```python
from build123d import *

# Parameters (mm, degrees)
EXTRU_MINCE3_DEPTH       = 85
EXTRU_MINCE4_DEPTH       = 14
ESQUISSE3_W              = 1
ESQUISSE3_H              = 39.023056592
EXTRU_MINCE5_DEPTH       = 14
ESQUISSE4_W              = 1
ESQUISSE4_H              = 39
EXTRU_MINCE6_DEPTH       = 14
ESQUISSE5_W              = 1
ESQUISSE5_H              = 37
EXTRU_MINCE7_DEPTH       = 14
ESQUISSE6_W              = 1
ESQUISSE6_H              = 37
EXTRU_MINCE8_DEPTH       = 14
ESQUISSE9_W              = 26
ESQUISSE9_H              = 39.023056592
ESQUISSE9_H_2            = 39
ESQUISSE9_W_2            = 27
BOSS_EXTRU_2_DEPTH       = 1
CONG_1_R                 = 10
CONG_2_R                 = 10
CONG_3_R                 = 10
CONG_4_R                 = 10
ESQUISSE10_W             = 23
ESQUISSE10_H             = 14
BOSS_EXTRU_3_DEPTH       = 3
ESQUISSE11_W             = 23
ESQUISSE11_H             = 14
BOSS_EXTRU_4_DEPTH       = 3
ESQUISSE14_R             = 1
ENL_V_MAT_EXTRU_2_DEPTH  = 15
ENL_V_START              = -15
ESQUISSE15_R             = 1
ENL_V_MAT_EXTRU_4_DEPTH  = 15
CHANFREIN2_SIZE2         = 1.154700538
CHANFREIN2_SIZE          = 2
CHANFREIN4_SIZE          = 2
CHANFREIN4_SIZE_2        = 2.22122503
BOSS_EXTRU_8_DEPTH       = 2
BOSS_EXTRU_9_DEPTH       = 2
ESQUISSE23_W             = 20
ESQUISSE23_H             = 10
ENL_V_MAT_EXTRU_7_DEPTH  = 2
ESQUISSE24_W             = 20
ESQUISSE24_H             = 10
ENL_V_MAT_EXTRU_9_DEPTH  = 2
ESQUISSE25_W             = 20
ESQUISSE25_H             = 10
ENL_V_MAT_EXTRU_11_DEPTH = 2
ESQUISSE26_W             = 20
ESQUISSE26_H             = 10
ENL_V_MAT_EXTRU_13_DEPTH = 2
ESQUISSE28_W             = 18
ESQUISSE28_H             = 4
R_VOL_MINCE9_ANGLE       = 50
ESQUISSE29_W             = 18
ESQUISSE29_H             = 4
R_VOL_MINCE10_ANGLE      = 50
ESQUISSE31_W             = 18
ESQUISSE31_H             = 4
R_VOL_MINCE11_ANGLE      = 50
ESQUISSE32_W             = 18
ESQUISSE32_H             = 4
R_VOL_MINCE12_ANGLE      = 50


# Some blends are built 0.0001 mm under size
with BuildPart() as part:
    # Esquisse1 → Extru.-Mince3 (new body)
    with BuildSketch(Plane.XY):
        Polygon((37.759483403, 45), (0, 0), (-200, 0), (-237.759483403, 45), (-236.227394517, 46.285575219), (-199.067384684, 2), (-0.932615316, 2), (36.227394517, 46.285575219), align=None)
    extrude(amount=EXTRU_MINCE3_DEPTH)

    # Esquisse2 → Extru.-Mince4 (add)
    with BuildSketch(Plane(origin=(0, 0, 0), x_dir=(-1, 0, 0), z_dir=(0, -1, 0))):
        Polygon((199.067384684, -46), (174, -46), (174, -85), (176, -85), (176, -48), (199.067384684, -48), align=None)
        Polygon((0, -48), (24, -48), (24, -85), (26, -85), (26, -46), (0, -46), align=None)
        Polygon((88.5, -85), (88.5, -48), (111.5, -48), (111.5, -85), (113.5, -85), (113.5, -46), (86.5, -46), (86.5, -85), align=None)
        Polygon((199.067384684, -37), (176, -37), (176, 0), (174, 0), (174, -39), (199.067384684, -39), align=None)
        Polygon((111.5, 0), (111.5, -37), (88.5, -37), (88.5, 0), (86.5, 0), (86.5, -39), (113.5, -39), (113.5, 0), align=None)
        Polygon((0, -39), (26, -39), (26, 0), (24, 0), (24, -37), (0, -37), align=None)
    extrude(amount=EXTRU_MINCE4_DEPTH)

    # Esquisse3 → Extru.-Mince5 (add)
    with BuildSketch(Plane(origin=(0, 0, 0), x_dir=(-1, 0, 0), z_dir=(0, -1, 0))):
        with Locations((199.5, -19.511528296)):
            Rectangle(ESQUISSE3_W, ESQUISSE3_H)
    extrude(amount=EXTRU_MINCE5_DEPTH)

    # Esquisse4 → Extru.-Mince6 (add)
    with BuildSketch(Plane.XZ):
        with Locations((-199.5, 65.5)):
            Rectangle(ESQUISSE4_W, ESQUISSE4_H)
    extrude(amount=EXTRU_MINCE6_DEPTH)

    # Esquisse5 → Extru.-Mince7 (add)
    with BuildSketch(Plane(origin=(0, 0, 0), x_dir=(-1, 0, 0), z_dir=(0, -1, 0))):
        with Locations((0.5, -18.5)):
            Rectangle(ESQUISSE5_W, ESQUISSE5_H)
    extrude(amount=EXTRU_MINCE7_DEPTH)

    # Esquisse6 → Extru.-Mince8 (add)
    with BuildSketch(Plane(origin=(0, 0, 0), x_dir=(-1, 0, 0), z_dir=(0, -1, 0))):
        with Locations((0.5, -66.5)):
            Rectangle(ESQUISSE6_W, ESQUISSE6_H)
    extrude(amount=EXTRU_MINCE8_DEPTH)

    # Esquisse9 → Boss.-Extru.2 (add)
    with BuildSketch(Plane(origin=(0, -14, 0), x_dir=(-1, 0, 0), z_dir=(0, -1, 0))):
        with Locations((187, -19.511528296)):
            Rectangle(ESQUISSE9_W, ESQUISSE9_H)
        with Locations((187, -65.5)):
            Rectangle(ESQUISSE9_W, ESQUISSE9_H_2)
        with Locations((100, -65.5)):
            Rectangle(ESQUISSE9_W_2, ESQUISSE9_H_2)
        with Locations((100, -19.5)):
            Rectangle(ESQUISSE9_W_2, ESQUISSE9_H_2)
        with Locations((13, -65.5)):
            Rectangle(ESQUISSE9_W, ESQUISSE9_H_2)
        with Locations((13, -19.5)):
            Rectangle(ESQUISSE9_W, ESQUISSE9_H_2)
    extrude(amount=BOSS_EXTRU_2_DEPTH)

    # Congé1
    cong_1_edges = [part.edges().sort_by_distance(p)[0] for p in [
        (-100, -15, 39),
    ]]
    fillet(cong_1_edges, radius=CONG_1_R)

    # Congé2
    cong_2_edges = [part.edges().sort_by_distance(p)[0] for p in [
        (-100, -14, 37),
    ]]
    fillet(cong_2_edges, radius=CONG_2_R)

    # Congé3
    cong_3_edges = [part.edges().sort_by_distance(p)[0] for p in [
        (-100, -15, 46),
    ]]
    fillet(cong_3_edges, radius=CONG_3_R)

    # Congé4
    cong_4_edges = [part.edges().sort_by_distance(p)[0] for p in [
        (-100, -14, 48),
    ]]
    fillet(cong_4_edges, radius=CONG_4_R)

    # Esquisse10 → Boss.-Extru.3 (add)
    with BuildSketch(Plane.XY.offset(85)):
        with Locations((-100, -7)):
            Rectangle(ESQUISSE10_W, ESQUISSE10_H)
    extrude(amount=-BOSS_EXTRU_3_DEPTH)

    # Esquisse11 → Boss.-Extru.4 (add)
    with BuildSketch(Plane(origin=(0, 0, 0), x_dir=(-1, 0, 0), z_dir=(0, 0, -1))):
        with Locations((100, -7)):
            Rectangle(ESQUISSE11_W, ESQUISSE11_H)
    extrude(amount=-BOSS_EXTRU_4_DEPTH)

    # Esquisse14 → Enlèv. mat.-Extru.2 (cut)
    with BuildSketch(Plane(origin=(0, 0, 0), x_dir=(-1, 0, 0), z_dir=(0, 0, -1))):
        with Locations((100, -6.5)):
            Circle(ESQUISSE14_R)
    extrude(amount=-ENL_V_MAT_EXTRU_2_DEPTH, mode=Mode.SUBTRACT)

    # Esquisse15 → Enlèv. mat.-Extru.4 (cut)
    with BuildSketch(Plane.XY.offset(85).offset(ENL_V_START)):
        with Locations(Location((-100, -6.5, 0), (0, 0, 180))):
            Circle(ESQUISSE15_R)
    extrude(amount=ENL_V_MAT_EXTRU_4_DEPTH, mode=Mode.SUBTRACT)

    # Chanfrein2
    chanfrein2_edges = [part.edges().sort_by_distance(p)[0] for p in [
        (36.227394517, 46.285575219, 42.5),
    ]]
    chanfrein2_side = [part.faces().sort_by_distance(p)[0] for p in [
        (36.245085555, 46.270730675, 42.5),
    ]]
    chamfer(chanfrein2_edges, length=CHANFREIN2_SIZE - 0.0001, length2=CHANFREIN2_SIZE2 - 0.0001, reference=chanfrein2_side[0])  # a hair under: the kernel refuses the full size

    # Chanfrein4
    # the kernel refuses this chamfer: 2.22122503, 2 mm, written as the material it takes off along each edge
    with BuildSketch(Plane(origin=(-236.227394517, 46.285575219, -5.720063061), x_dir=(0.6670048935936307, -0.7450533349513642, 0), z_dir=(0, 0, 1))) as chanfrein4_piece_1:
        Polygon((CHANFREIN4_SIZE * 0.999486448269, -CHANFREIN4_SIZE * 0.0320443400082), (-CHANFREIN4_SIZE_2 * 0.0320443400033, -CHANFREIN4_SIZE_2 * 0.999486448115), (0, 0), align=None)
    extrude(amount=96.440126123, mode=Mode.SUBTRACT)

    # Esquisse17 → Boss.-Extru.8 (add)
    with BuildSketch(Plane.XY.offset(85)):
        Polygon((35.485167318, 45.401023288), (-235.485167318, 45.401023288), (-199.067384684, 2), (-0.932615316, 2), align=None)
    extrude(amount=-BOSS_EXTRU_8_DEPTH)

    # Esquisse18 → Boss.-Extru.9 (add)
    with BuildSketch(Plane(origin=(0, 0, 0), x_dir=(-1, 0, 0), z_dir=(0, 0, -1))):
        Polygon((-35.485167318, 45.401023288), (235.485167318, 45.401023288), (199.067384684, 2), (0.932615316, 2), align=None)
    extrude(amount=-BOSS_EXTRU_9_DEPTH)

    # Esquisse23 → Enlèv. mat.-Extru.7 (cut)
    with BuildSketch(Plane(origin=(0, 0, 0), x_dir=(-1, 0, 0), z_dir=(0, -1, 0))):
        with Locations((13.5, -32)):
            Rectangle(ESQUISSE23_W, ESQUISSE23_H)
    extrude(amount=-ENL_V_MAT_EXTRU_7_DEPTH, mode=Mode.SUBTRACT)

    # Esquisse24 → Enlèv. mat.-Extru.9 (cut)
    with BuildSketch(Plane.XZ):
        with Locations((-13.5, 53)):
            Rectangle(ESQUISSE24_W, ESQUISSE24_H)
    extrude(amount=-ENL_V_MAT_EXTRU_9_DEPTH, mode=Mode.SUBTRACT)

    # Esquisse25 → Enlèv. mat.-Extru.11 (cut)
    with BuildSketch(Plane(origin=(0, 0, 0), x_dir=(-1, 0, 0), z_dir=(0, -1, 0))):
        with Locations((186.5, -53)):
            Rectangle(ESQUISSE25_W, ESQUISSE25_H)
    extrude(amount=-ENL_V_MAT_EXTRU_11_DEPTH, mode=Mode.SUBTRACT)

    # Esquisse26 → Enlèv. mat.-Extru.13 (cut)
    with BuildSketch(Plane(origin=(0, 0, 0), x_dir=(-1, 0, 0), z_dir=(0, -1, 0))):
        with Locations((186.5, -32)):
            Rectangle(ESQUISSE26_W, ESQUISSE26_H)
    extrude(amount=-ENL_V_MAT_EXTRU_13_DEPTH, mode=Mode.SUBTRACT)

    # Esquisse28 → Révol.-Mince9 (revolve)
    with BuildSketch(Plane(origin=(-115.83272888, -97.195200082, 0), x_dir=(0, 0, -1), z_dir=(0.7660444431189792, 0.6427876096865379, 0))):
        with Locations((-74.044453546, 153.490137254)):
            Rectangle(ESQUISSE28_W, ESQUISSE28_H)
    revolve(axis=Axis((-215.779862536, 21.917155521, 83.044453546), (0, 0, 1)), revolution_arc=R_VOL_MINCE9_ANGLE)

    # Esquisse29 → Révol.-Mince10 (revolve)
    with BuildSketch(Plane(origin=(-115.83272888, -97.195200082, 0), x_dir=(0, 0, -1), z_dir=(0.7660444431189792, 0.6427876096865379, 0))):
        with Locations((-11, 153.490137254)):
            Rectangle(ESQUISSE29_W, ESQUISSE29_H)
    revolve(axis=Axis((-215.779862536, 21.917155521, 2), (0, 0, 1)), revolution_arc=R_VOL_MINCE10_ANGLE)

    # Esquisse31 → Révol.-Mince11 (revolve)
    with BuildSketch(Plane(origin=(-1.532088886, 1.285575219, 0), x_dir=(0, 0, 1), z_dir=(-0.7660444431189749, 0.642787609686543, 0))):
        with Locations((11, 24.932615316)):
            Rectangle(ESQUISSE31_W, ESQUISSE31_H)
    revolve(axis=Axis((15.779862536, 21.917155521, 2), (0, 0, -1)), revolution_arc=R_VOL_MINCE11_ANGLE)

    # Esquisse32 → Révol.-Mince12 (revolve)
    with BuildSketch(Plane(origin=(-1.532088886, 1.285575219, 0), x_dir=(0, 0, 1), z_dir=(-0.7660444431189749, 0.642787609686543, 0))):
        with Locations((74, 24.932615316)):
            Rectangle(ESQUISSE32_W, ESQUISSE32_H)
    revolve(axis=Axis((15.779862536, 21.917155521, 83), (0, 0, -1)), revolution_arc=R_VOL_MINCE12_ANGLE)


solid = part.part
```
Input: part model. Units: mm. Frame: model coordinates. A direction names the side the tool comes from. Give positions to 0.01 mm unless a question says otherwise; leave off trailing zeros. Order: outer loops, then holes, each group sorted by start corner. A loop starts at its lowest first (then second) coordinate and runs counter-clockwise, first axis right, second up.
1. Section D-D on z = 73. Give the number of separate pieces and of enclosed holes in the cut face, and give its area (3 significant figures).
Derived:
separate pieces: 1
enclosed holes: 3
area: 861 mm2
2. Pin query (flat end, axial travel): pin 1 (1.6 mm diameter, centred on y = 1, z = 52, fed in from -X); pin 2 (0.6 mm diameter, centred on y = 1, z = 51.5, fed in from -X); pin 3 (11 mm diameter, centred on y = -6.5, z = 73.5, fed in from +X). Return the tip coordinate at first contact, or that it passes through.
Derived:
pin 1: stops at x = -201.51
pin 2: stops at x = -201.09
pin 3: stops at x = 0
3. Mould query, pull axis Y, two halves, no side actions, for faces 1 (the flat face through (-199, -7, 66)), 2 (the flat face through (-111.5, -7, 65)), 3 (the cylindrical face through (-100.19, -11.99, 48.85)), 4 (the flat face through (0, -7, 20)). Classes: released by +Y, released by -Y, zero draft, split by the parting line, or undercut.
Derived:
face 1: undercut
face 2: undercut
face 3: released by -Y
face 4: zero draft
4. Section A-A on x = -92. Return the cut outline in (y, z), and give its area (3 significant figures).
Derived:
outline: (-15, 0) - (45.4, 0) - (45.4, 2) - (2, 2) - (2, 83) - (45.4, 83) - (45.4, 85) - (-15, 85) - (-15, 56) arc R10 ccw to (-5, 46) - (0, 46) - (0, 39) - (-5, 39) arc R10 ccw to (-15, 29) - close; hole (-14, 3) - (0, 3) - (0, 37) - (-4, 37) arc R10 ccw to (-14, 27) - close; hole (-14, 58) arc R10 ccw to (-4, 48) - (0, 48) - (0, 82) - (-14, 82) - close
area: 562 mm2
5. Material intervals for L1, parallel to X at y = -5, z = 63.5; L2, parallel to Y at x = -100, z = 1.55; L3, parallel to Z at x = -178.5, y = 19, sorted ascending.
Derived:
L1: x = -200 to -199, -176 to -174, -113.5 to -111.5, -88.5 to -86.5, -26 to -24, -1 to 0
L2: y = -15 to -7.5, -5.5 to 45.4
L3: z = 0 to 2, 83 to 85
6. Reachability of faces 5 (the flat face through (-100, -2, 39)), 6 (the flat face through (-100, -5, 3)), 7 (the flat face through (-24, -7, 66)), 8 (the flat face through (0, -7, 66)) from +Z, -Z, +X, -X, +Y, -Y: full face, straight path, thin tool, end or side. Return the list, or none.
Derived:
face 5: +X, -X, -Y
face 6: none
face 7: +Z
face 8: +Z, -Z, +X, -Y
7. Section C-C on x = -159. Return the cut outline in (y, z), and give its area (3 significant figures).
Derived:
outline: (0, 0) - (45.4, 0) - (45.4, 2) - (2, 2) - (2, 83) - (45.4, 83) - (45.4, 85) - (0, 85) - close
area: 344 mm2
8. Section B-B on y = 10. Return the cut outline in (x, z), and give its area (3 significant figures).
Derived:
outline: (-208.39, 0) - (8.39, 0) - (8.39, 85) - (-208.39, 85) - close; hole (-205.78, 2) - (5.78, 2) - (5.78, 83) - (-205.78, 83) - close
area: 1,290 mm2
